```python
from build123d import *

# Parameters (mm, degrees)
SKETCH1_W           = 71.12
SKETCH1_H           = 30.48
BOSS_EXTRUDE1_DEPTH = 14.732
SKETCH2_R           = 4.191
CUT_EXTRUDE1_DEPTH  = 12.7
CUT_EXTRUDE2_START  = -25.4
SKETCH3_R           = 4.191
CUT_EXTRUDE2_DEPTH  = 25.4
SKETCH4_W           = 14.732
SKETCH4_H           = 5.08
SKETCH4_W_2         = 6.35
SKETCH4_H_2         = 8.128
SKETCH4_W_3         = 20.066
CUT_EXTRUDE3_DEPTH  = 1.3335
BOSS_EXTRUDE2_DEPTH = 1.905
BOSS_EXTRUDE3_DEPTH = 1.905
SKETCH7_W           = 14.732
SKETCH7_H           = 5.08
SKETCH7_W_2         = 20.066
SKETCH7_H_2         = 8.128
SKETCH7_W_3         = 6.35
CUT_EXTRUDE4_DEPTH  = 1.3335


with BuildPart() as part:
    # Sketch1 → Boss-Extrude1 (new body)
    with BuildSketch(Plane(origin=(0, 0, 0), x_dir=(1, 0, 0), z_dir=(0, 1, 0))):
        with Locations((35.56, 15.24)):
            Rectangle(SKETCH1_W, SKETCH1_H)
    extrude(amount=BOSS_EXTRUDE1_DEPTH)

    # Sketch2 → Cut-Extrude1 (cut)
    with BuildSketch(Plane(origin=(71.12, 0, 0), x_dir=(0, 0, -1), z_dir=(1, 0, 0))):
        with Locations((15.24, 7.493)):
            Circle(SKETCH2_R)
        with Locations((25.019, 7.493)):
            Circle(SKETCH2_R)
        with Locations((5.461, 7.493)):
            Circle(SKETCH2_R)
    extrude(amount=-CUT_EXTRUDE1_DEPTH, mode=Mode.SUBTRACT)

    # Sketch3 → Cut-Extrude2 (cut)
    with BuildSketch(Plane.ZY.offset(CUT_EXTRUDE2_START)):
        with Locations(Location((-15.24, 7.493, 0), (0, 0, 180))):
            Circle(SKETCH3_R)
        with Locations(Location((-5.461, 7.493, 0), (0, 0, 180))):
            Circle(SKETCH3_R)
        with Locations(Location((-25.019, 7.493, 0), (0, 0, 180))):
            Circle(SKETCH3_R)
    extrude(amount=CUT_EXTRUDE2_DEPTH, mode=Mode.SUBTRACT)

    # Sketch4 → Cut-Extrude3 (cut)
    with BuildSketch(Plane(origin=(0, 14.732, 0), x_dir=(1, 0, 0), z_dir=(0, 1, 0))):
        with Locations((63.754, 20.447)):
            Rectangle(SKETCH4_W, SKETCH4_H)
        with Locations((63.754, 10.033)):
            Rectangle(SKETCH4_W, SKETCH4_H)
        with Locations((48.641, 20.574)):
            Rectangle(SKETCH4_W_2, SKETCH4_H_2)
        with Locations((48.641, 9.906)):
            Rectangle(SKETCH4_W_2, SKETCH4_H_2)
        with Locations((29.337, 20.574)):
            Rectangle(SKETCH4_W_3, SKETCH4_H_2)
        with Locations((29.337, 9.906)):
            Rectangle(SKETCH4_W_3, SKETCH4_H_2)
        with Locations((7.366, 20.447)):
            Rectangle(SKETCH4_W, SKETCH4_H)
        with Locations((7.366, 10.033)):
            Rectangle(SKETCH4_W, SKETCH4_H)
    extrude(amount=-CUT_EXTRUDE3_DEPTH, mode=Mode.SUBTRACT)

    # Sketch5 → Boss-Extrude2 (add)
    with BuildSketch(Plane.XY):
        Polygon((60.452, 3.8735), (60.452, 10.8585), (57.785, 10.8585), (56.769, 9.906), (56.769, 4.826), (57.785, 3.8735), align=None)
        Polygon((13.843, 3.8735), (11.176, 3.8735), (11.176, 10.8585), (13.843, 10.8585), (14.859, 9.906), (14.859, 4.826), align=None)
    extrude(amount=BOSS_EXTRUDE2_DEPTH)

    # Sketch6 → Boss-Extrude3 (add)
    with BuildSketch(Plane(origin=(0, 0, -30.48), x_dir=(-1, 0, 0), z_dir=(0, 0, -1))):
        Polygon((-60.452, 11.938), (-60.452, 2.794), (-57.785, 2.794), (-56.769, 3.937), (-56.769, 10.795), (-57.785, 11.938), align=None)
        Polygon((-13.335, 11.938), (-10.668, 11.938), (-10.668, 2.794), (-13.335, 2.794), (-14.351, 3.937), (-14.351, 10.795), align=None)
    extrude(amount=BOSS_EXTRUDE3_DEPTH)

    # Sketch7 → Cut-Extrude4 (cut)
    with BuildSketch(Plane.XZ):
        with Locations((7.366, -20.447)):
            Rectangle(SKETCH7_W, SKETCH7_H)
        with Locations((7.366, -10.033)):
            Rectangle(SKETCH7_W, SKETCH7_H)
        with Locations((29.337, -20.574)):
            Rectangle(SKETCH7_W_2, SKETCH7_H_2)
        with Locations((29.337, -9.906)):
            Rectangle(SKETCH7_W_2, SKETCH7_H_2)
        with Locations((48.641, -20.574)):
            Rectangle(SKETCH7_W_3, SKETCH7_H_2)
        with Locations((48.641, -9.906)):
            Rectangle(SKETCH7_W_3, SKETCH7_H_2)
        with Locations((63.754, -20.447)):
            Rectangle(SKETCH7_W, SKETCH7_H)
        with Locations((63.754, -10.033)):
            Rectangle(SKETCH7_W, SKETCH7_H)
    extrude(amount=-CUT_EXTRUDE4_DEPTH, mode=Mode.SUBTRACT)


solid = part.part
```
Work out the finished part from the listing and answer in its coordinate system (mm). A direction names the side the tool comes from. Coordinates: 2 decimals unless noted, no trailing zeros. Order: outer loops, then holes, each group sorted by start corner. A loop starts at its lowest first (then second) coordinate and runs counter-clockwise, first axis right, second up. Notation, with made-up numbers: (36, 55) - (67, 55) arc R20 ccw to (67, 76) - close; hole circle Ø6 at (77, 38.25). An arc over 180 degrees is marked (long way). Answer as a JSON object with one key per item and string values.
1. A tool of negligible diameter and unlimited length cuts with its end or side. For faces 4 (the face through (64, 1, -17.907)), 5 (the face through (7, 1.334, -10)), 6 (the face through (49, 14, -24.638)), 7 (the face through (49, 1, -16.51)), 8 (the face through (11.176, 7, 1)), from which of +Z, -Z, +X, -X, +Y, -Y can it reach the whole face along a straight path? Write none if from no direction.
Output values:
{"face 4": "+X, -Y", "face 5": "-X, -Y", "face 6": "+Y", "face 7": "-Y", "face 8": "+Z, -X, +Y, -Y"}
2. Find section C-C on z = -5. Determine the outline of the cut face in (x, y), plus the area to 3 significant figures.
Output values:
{"outline": "(0, 0) - (71.12, 0) - (71.12, 3.33) - (58.42, 3.33) - (58.42, 11.66) - (71.12, 11.66) - (71.12, 14.73) - (0, 14.73) - (0, 11.66) - (25.4, 11.66) - (25.4, 3.33) - (0, 3.33) - close", "area": "730 mm²"}
3. Consider line 1 (X direction, y = 13.75, z = -6.5); line 2 (X direction, y = 1.25, z = -10.5); line 3 (Z direction, x = 32.5, y = 14). Determine where each line is inside the solid, lowest interval first.
Output values:
{"line 1": "x = 0 to 19.3, 39.37 to 45.47, 51.82 to 71.12", "line 2": "x = 14.73 to 19.3, 39.37 to 45.47, 51.82 to 56.39", "line 3": "z = -30.48 to -24.64, -16.51 to -13.97, -5.84 to 0"}
4. Each of these flat-tipped pins is pushed along its axis until it touches: P1, Ø2, axis at x = 49.5, z = -21, coming from the +Y side; P2, Ø1.1, axis at x = 47, y = 14, coming from the -Z side; P3, Ø1.5, axis at y = 14.5, z = -19.5, coming from the +X side. Where does it stop, or does it pass through?
Output values:
{"P1": "stops at y = 13.4", "P2": "stops at z = -30.48", "P3": "stops at x = 56.39"}
5. Find section A-A on z = -15.24. Determine the outline of the cut face in (x, y).
Output values:
{"outline": "(0, 0) - (71.12, 0) - (71.12, 3.3) - (58.42, 3.3) - (58.42, 11.68) - (71.12, 11.68) - (71.12, 14.73) - (0, 14.73) - (0, 11.68) - (25.4, 11.68) - (25.4, 3.3) - (0, 3.3) - close"}
6. The mould has two halves that part along X. Classify faces 1 (the face through (71.12, 4, -12)), 2 (the face through (64, 1.334, -10)), 3 (the face through (39.37, 14, -10)): +X half, -X half, draft (parallel to the pull), parting line (faces both ways), or undercut.
Output values:
{"face 1": "+X half", "face 2": "draft", "face 3": "undercut"}
7. Find section B-B on x = 34. Determine the outline of the cut face in (y, z), plus the area to 3 significant figures.
Output values:
{"outline": "(0, -30.48) - (14.73, -30.48) - (14.73, -24.64) - (13.4, -24.64) - (13.4, -16.51) - (14.73, -16.51) - (14.73, -13.97) - (13.4, -13.97) - (13.4, -5.84) - (14.73, -5.84) - (14.73, 0) - (0, 0) - (0, -5.84) - (1.33, -5.84) - (1.33, -13.97) - (0, -13.97) - (0, -16.51) - (1.33, -16.51) - (1.33, -24.64) - (0, -24.64) - close", "area": "406 mm²"}
